Work out the finished part from the listing and answer in its coordinate system (mm). Round coordinates to 2 decimals unless told otherwise and drop trailing zeros. Write each loop counter-clockwise with the first axis right and the second up, starting at its lowest first coordinate (ties: lowest second). Pieces come first, ordered by that corner, then holes. Notation, with made-up numbers: (31.25, -14.5) - (73.25, -14.5) arc R29 cw to (73.25, 22.5) - close; hole circle Ø8 at (84.5, 65). An arc over 180 degrees is marked (long way). Answer as a JSON object with one key per item and string values.
```python
from build123d import *

# Parameters (mm, degrees)
BOSS_EXTRUDE1_DEPTH = 5
SKETCH2_R           = 5
SKETCH2_R_2         = 2.5
SKETCH2_R_3         = 4
SKETCH2_R_4         = 2
SKETCH2_R_5         = 1.5
CUT_EXTRUDE1_DEPTH  = 10


with BuildPart() as part:
    # Sketch1 → Boss-Extrude1 (new body)
    with BuildSketch(Plane(origin=(0, 0, 0), x_dir=(1, 0, 0), z_dir=(0, 1, 0))):
        with BuildLine():
            Line((-175, 48), (175, 48))
            ThreePointArc((175, 48), (223, 0), (175, -48))
            Line((175, -48), (-175, -48))
            ThreePointArc((-175, -48), (-223, 0), (-175, 48))
        make_face()
    extrude(amount=BOSS_EXTRUDE1_DEPTH)

    # Sketch2 → Cut-Extrude1 (cut)
    with BuildSketch(Plane.XZ):
        with Locations(Location((175, 0, 0), (0, 0, 270))):
            Circle(SKETCH2_R)
        with Locations(Location((175, 18.65, 0), (0, 0, 270))):
            Circle(SKETCH2_R_2)
        with Locations(Location((175, -18.65, 0), (0, 0, 270))):
            Circle(SKETCH2_R_2)
        with Locations(Location((-175, -18.65, 0), (0, 0, 90))):
            Circle(SKETCH2_R_2)
        with Locations(Location((-175, 18.65, 0), (0, 0, 90))):
            Circle(SKETCH2_R_2)
        with Locations(Location((-175, 0, 0), (0, 0, 270))):
            Circle(SKETCH2_R)
        with Locations(Location((120, 0, 0), (0, 0, 270))):
            Circle(SKETCH2_R_3)
        with Locations(Location((95.25, -14.7, 0), (0, 0, 270))):
            Circle(SKETCH2_R_4)
        with Locations(Location((144.75, -14.7, 0), (0, 0, 270))):
            Circle(SKETCH2_R_4)
        with Locations(Location((144.75, 34.8, 0), (0, 0, 270))):
            Circle(SKETCH2_R_4)
        with Locations(Location((95.25, 34.8, 0), (0, 0, 270))):
            Circle(SKETCH2_R_4)
        with Locations(Location((-135.5, -15.5, 0), (0, 0, 270))):
            Circle(SKETCH2_R_5)
        with Locations(Location((-135.5, 15.5, 0), (0, 0, 270))):
            Circle(SKETCH2_R_5)
        with Locations(Location((-104.5, 15.5, 0), (0, 0, 270))):
            Circle(SKETCH2_R_5)
        with Locations(Location((-104.5, -15.5, 0), (0, 0, 270))):
            Circle(SKETCH2_R_5)
        with Locations(Location((-120, 0, 0), (0, 0, 270))):
            Circle(SKETCH2_R_2)
    extrude(amount=-CUT_EXTRUDE1_DEPTH, mode=Mode.SUBTRACT)


solid = part.part
```
Item 1: A cutting plane is placed at C-C (z = -41). Write down the section's boundary in (x, y), and give its area (3 significant figures).
Results found:
{"outline": "(-199.96, 0) - (199.96, 0) - (199.96, 5) - (-199.96, 5) - close", "area": "2,000 mm²"}
Item 2: Each of these flat-tipped pins is pushed along its axis until it touches: P1, Ø2, axis at y = 2, z = -8.5, coming from the +X side; P2, Ø1.5, axis at y = 2.5, z = -33, coming from the -X side; P3, Ø3, axis at y = 4, z = -13.5, coming from the +X side. Where does it stop, or does it pass through?
Results found:
{"P1": "x = 222.41", "P2": "x = -210.55", "P3": "x = 221.48"}
Item 3: A cutting plane is placed at A-A (y = 3.15). Give the number of separate pieces and of enclosed holes in the cut face, and give its area (3 significant figures).
Results found:
{"separate pieces": "1", "enclosed holes": "16", "area": "40,500 mm²"}
Item 4: A cutting plane is placed at B-B (z = 42). Write down the section's boundary in (x, y).
Results found:
{"outline": "(-198.24, 0) - (198.24, 0) - (198.24, 5) - (-198.24, 5) - close"}
Item 5: Determine the mould class of faces 1 (the cylindrical face through (-170.043, 2.465, 0.651)), 2 (the cylindrical face through (123.966, 2.465, 0.521)), 3 (the cylindrical face through (222.99, 2.46, -1.06)), 4 (the flat face through (3, 0, -1)) for opening direction Z: pulls with the +Z half, pulls with the -Z half, needs draft (parallel to the pull), parting line crosses it, or undercut.
Results found:
{"face 1": "undercut", "face 2": "undercut", "face 3": "parting line crosses it", "face 4": "needs draft"}
Item 6: Consider line 1 along Z through (x, y) = (-135.5, 2.05); line 2 along X through (y, z) = (3.8, 36.5); line 3 along X through (y, z) = (2.2, -18.65). Determine where each line is inside the solid, lowest interval first.
Results found:
{"line 1": "-48 to -17, -14 to 14, 17 to 48", "line 2": "-206.17 to 94.2, 96.3 to 143.7, 145.8 to 206.17", "line 3": "-219.23 to -177.5, -172.5 to 172.5, 177.5 to 219.23"}
